Part print with two shaded views. Sizes in mm from the minimum x, y, z corner. A direction names the side the tool comes from. Round coordinates to 2 decimals unless told otherwise and drop trailing zeros. Loops run counter-clockwise (first coordinate to the right, second up) from the corner with the lowest first, then second, coordinate; pieces in that order, holes last. Notation, with made-up numbers: (-32.5, 58.25) - (-15.5, 58.25) arc R23 cw to (-15.5, 73.25) - close; hole circle Ø3 at (-10.75, -21.5). An arc over 180 degrees is marked (long way). One line per question, with ' | ' between items.
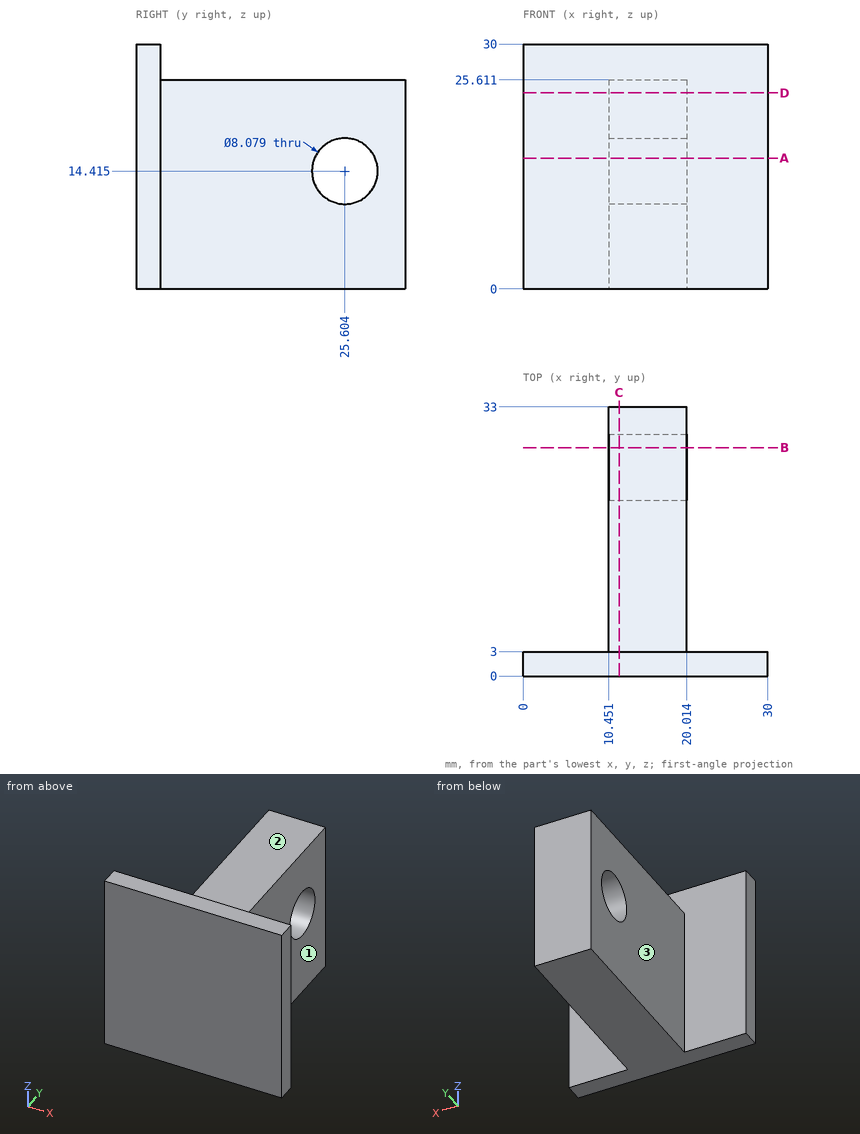
(1) Cut at C-C, the plane x = 11.75. Write the cut outline in (y, z) (1 decimal), then the cut area to 3 significant figures.
Results found:
outline: (0, 0) - (33, 0) - (33, 25.6) - (3, 25.6) - (3, 30) - (0, 30) - close; hole circle Ø8.1 at (25.6, 14.4) | area: 807 mm²
(2) Cut at D-D, the plane z = 24. Write the cut outline in (x, y).
Results found:
outline: (0, 0) - (30, 0) - (30, 3) - (20.01, 3) - (20.01, 33) - (10.45, 33) - (10.45, 3) - (0, 3) - close
(3) Drop flat-ended pins along their axis: P1, Ø2, axis at y = 12.5, z = 11.5, coming from the -X side; P2, Ø13, axis at y = 21, z = 18.5, coming from the +X side; P3, Ø6, axis at x = 7, z = 12.5, coming from the +Y side. Give the stop position or say it passes through.
Results found:
P1: stops at x = 10.45 | P2: stops at x = 20.01 | P3: stops at y = 3
(4) Probe L1, parallel to Y at x = 28.25, z = 1.5; L2, parallel to X at y = 29.5, z = 25.5; L3, parallel to Z at x = 19.5, y = 5.5. List the from-to ranges inside material, lowest first.
Results found:
L1: y = 0 to 3 | L2: x = 10.45 to 20.01 | L3: z = 0 to 25.61
(5) Tool access for the marked faces 1, 2 and 3: list every direction of +Z, -Z, +X, -X, +Y, -Y with a clear straight run to the whole face (end or side of a thin tool).
Results found:
face 1: +Z, -Z, +X, +Y | face 2: +Z, +X, -X, +Y | face 3: +Z, -Z, -X, +Y
(6) Cut at A-A, the plane z = 16. Write the cut outline in (x, y).
Results found:
outline: (0, 0) - (30, 0) - (30, 3) - (20.01, 3) - (20.01, 21.89) - (10.45, 21.89) - (10.45, 3) - (0, 3) - close; (10.45, 29.32) - (20.01, 29.32) - (20.01, 33) - (10.45, 33) - close
(7) Cut at B-B, the plane y = 28. Write the cut outline in (x, z), then the cut area to 3 significant figures.
Results found:
outline: (10.45, 0) - (20.01, 0) - (20.01, 11.16) - (10.45, 11.16) - close; (10.45, 17.67) - (20.01, 17.67) - (20.01, 25.61) - (10.45, 25.61) - close | area: 183 mm²
